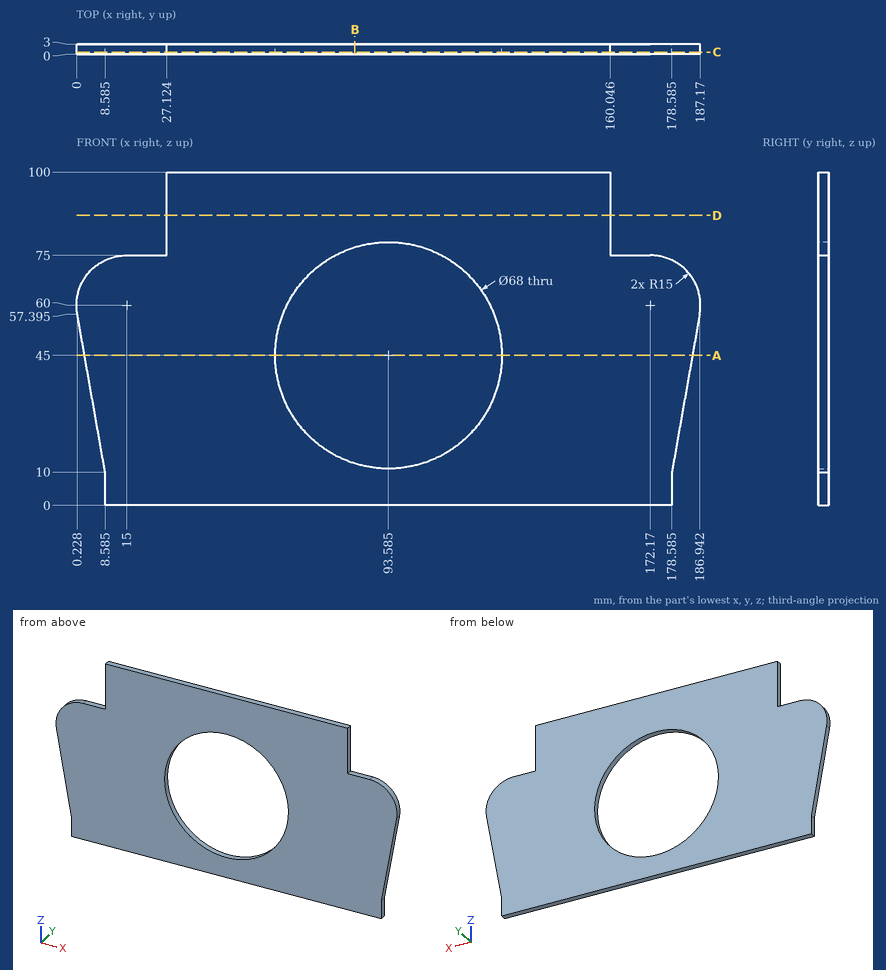
Can you work these out from the drawing? Everything is in mm from the part's minimum corner. Coordinates: 2 decimals unless noted, no trailing zeros. Loops run counter-clockwise (first coordinate to the right, second up) from the corner with the lowest first, then second, coordinate; pieces in that order, holes last. Notation, with made-up numbers: (70, 83) - (128, 83) arc R26 ccw to (128, 105) - close; hole circle Ø10 at (13, 56.5). An arc over 180 degrees is marked (long way). Answer as CSV lines item,"result".
Q1. If I drill on L1, parallel to X at y = 1.45, z = 65; L2, parallel to Z at x = 114.5, y = 2.45 (1 decimal); L3, parallel to X at y = 2, z = 45 (1 decimal), over which ranges is the centre line in solid material (lowest first)? Write a range as [from, to].
Response:
L1,"[0.86, 66.09], [121.08, 186.31]"
L2,"[0, 18.2], [71.8, 100]"
L3,"[2.4, 59.6], [127.6, 184.8]"
Q2. If we section it at A-A, the plane z = 45: Write out the boundary of the cut face in (x, y) (1 decimal).
Response:
outline,"(2.4, 0) - (59.6, 0) - (59.6, 3) - (2.4, 3) - close; (127.6, 0) - (184.8, 0) - (184.8, 3) - (127.6, 3) - close"
Q3. For pin 1 (0.9 mm diameter, centred on y = 2, z = 91, fed in from +X); pin 2 (1.5 mm diameter, centred on x = 166, y = 1, fed in from +Z); pin 3 (0.9 mm diameter, centred on y = 2, z = 4.5, fed in from +X) (3 decimals), each with a flat end and sliding along its axis, tell me the tip position at first contact or that it passes through.
Response:
pin 1,"x = 160.05"
pin 2,"z = 75"
pin 3,"x = 178.585"
Q4. If we section it at C-C, the plane y = 0.6: Write out the boundary of the cut face in (x, z) (1 decimal).
Response:
outline,"(0.2, 57.4) - (8.6, 10) - (8.6, 0) - (178.6, 0) - (178.6, 10) - (186.9, 57.4) arc R15 ccw to (172.2, 75) - (160, 75) - (160, 100) - (27.1, 100) - (27.1, 75) - (15, 75) arc R15 ccw to start; hole circle Ø68 at (93.6, 45)"
Q5. If we section it at D-D, the plane z = 87: Write out the boundary of the cut face in (x, y), and give its area (3 significant figures).
Response:
outline,"(27.12, 0) - (160.05, 0) - (160.05, 3) - (27.12, 3) - close"
area,"399 mm2"
Q6. If we section it at B-B, the plane x = 83.5: Write out the boundary of the cut face in (y, z).
Response:
outline,"(0, 0) - (3, 0) - (3, 12.53) - (0, 12.53) - close; (0, 77.47) - (3, 77.47) - (3, 100) - (0, 100) - close"
